Verification items for the finished model (mm, model axes). A direction names the side the tool comes from. Coordinates: 2 decimals unless noted, no trailing zeros. Order: outer loops, then holes, each group sorted by start corner. A loop starts at its lowest first (then second) coordinate and runs counter-clockwise, first axis right, second up.
Q1. Thickness scan on line 1 (Y direction, x = 0, z = 2.65); line 2 (X direction, y = 0, z = 63); line 3 (Z direction, x = 1.75, y = 3.5). Record the ranges inside material, lowest first.
Q2. Depth check by flat-ended pin: P1, Ø2, axis at x = 5.5, y = 1.5, coming from the +Z side; P2, Ø3, axis at x = 0, y = 0, coming from the -Z side. Enter the tip coordinate at first touch or a pass-through.
Q3. Set-up check for faces 4 (the cylindrical face through (0.54, -2.44, 2.46)), 5 (the flat face through (2, 2, 15)), 6 (the cylindrical face through (7, 6, 60)): record each of +Z, -Z, +X, -X, +Y, -Y from which the full face is reachable in a straight line by a thin tool's end or side.
Q4. Draft check along X on faces 1 (the flat face through (2, 2, 70)), 2 (the flat face through (12.128, 12.086, 62.03)), 3 (the flat face through (0, 0, 5)). Enter one of: pulls with the +X half, pulls with the -X half, needs draft (parallel to the pull), parting line crosses it, or undercut.
Q5. Cross-section at A-A, the plane z = 56. Record the boundary of the cut face in (x, y).
from build123d import *

# Parameters (mm, degrees)
ESQUISSE1_R             = 3
BOSS_EXTRU_1_DEPTH      = 15
ESQUISSE2_R             = 2.5
ENL_V_MAT_EXTRU_1_DEPTH = 5
BOSS_EXTRU_2_DEPTH      = 55
ESQUISSE4_R             = 2.121320344
BOSS_EXTRU_3_DEPTH      = 15
ESQUISSE5_R             = 3
BOSS_EXTRU_4_DEPTH      = 30


with BuildPart() as part:
    # Esquisse1 → Boss.-Extru.1 (new body)
    with BuildSketch(Plane.XY):
        Circle(ESQUISSE1_R)
    extrude(amount=BOSS_EXTRU_1_DEPTH)

    # Esquisse2 → Enlèv. mat.-Extru.1 (cut)
    with BuildSketch(Plane(origin=(0, 0, 0), x_dir=(-1, 0, 0), z_dir=(0, 0, -1))):
        Circle(ESQUISSE2_R)
    extrude(amount=-ENL_V_MAT_EXTRU_1_DEPTH, mode=Mode.SUBTRACT)

    # Esquisse3 → Boss.-Extru.2 (add)
    with BuildSketch(Plane.XY.offset(15)):
        with BuildLine():
            Line((0, 3), (3, 0))
            ThreePointArc((3, 0), (-2.121320344, -2.121320344), (0, 3))
        make_face()
    extrude(amount=BOSS_EXTRU_2_DEPTH)

    # Esquisse4 → Boss.-Extru.3 (add)
    with BuildSketch(Plane(origin=(1.5, 1.5, 0), x_dir=(0, 0, -1), z_dir=(0.7071067811865477, 0.7071067811865475, 0))):
        with Locations(Location((-62, 0, 0), (0, 0, 90))):
            Circle(ESQUISSE4_R)
        with Locations(Location((-32, 0, 0), (0, 0, 90))):
            Circle(ESQUISSE4_R)
    extrude(amount=BOSS_EXTRU_3_DEPTH)

    # Esquisse5 → Boss.-Extru.4 (add)
    with BuildSketch(Plane.XY.offset(70)):
        Circle(ESQUISSE5_R)
    extrude(amount=BOSS_EXTRU_4_DEPTH)


solid = part.part
Check values:
1. line 1: y = -3 to -2.5, 2.5 to 3
1. line 2: x = -3 to 3
1. line 3: z = 30.28 to 33.72, 60.28 to 63.72
2. P1: stops at z = 63.08
2. P2: stops at z = 5
3. face 4: -Z
3. face 5: +X, +Y
3. face 6: none
4. face 1: needs draft
4. face 2: pulls with the +X half
4. face 3: undercut
5. outline: (0, 3) arc R3 ccw (long way) to (3, 0) - close
